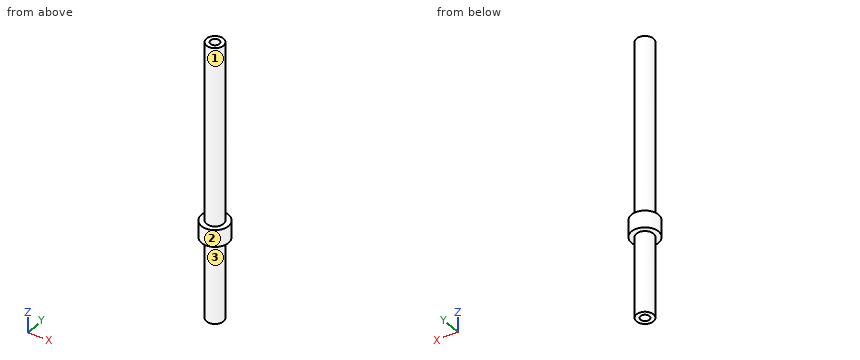
from build123d import *

# Parameters (mm, degrees)
SKETCH1_R                 = 2.5
BOSS_EXTRUDE1_DEPTH       = 24
SKETCH2_R                 = 4
BOSS_EXTRUDE2_DEPTH       = 5
SKETCH3_R                 = 2.5
BOSS_EXTRUDE3_DEPTH       = 53
M3X0_5_TAPPED_HOLE1_D     = 2.6
M3X0_5_TAPPED_HOLE1_DEPTH = 8
M3X0_5_TAPPED_HOLE1_TIP   = 0.781118805
M3X0_5_TAPPED_HOLE2_D     = 2.6
M3X0_5_TAPPED_HOLE2_DEPTH = 8
M3X0_5_TAPPED_HOLE2_TIP   = 0.781118805


with BuildPart() as part:
    # Sketch1 → Boss-Extrude1 (new body)
    with BuildSketch(Plane.XY):
        Circle(SKETCH1_R)
    extrude(amount=BOSS_EXTRUDE1_DEPTH)

    # Sketch2 → Boss-Extrude2 (add)
    with BuildSketch(Plane.XY.offset(24)):
        Circle(SKETCH2_R)
    extrude(amount=BOSS_EXTRUDE2_DEPTH)

    # Sketch3 → Boss-Extrude3 (add)
    with BuildSketch(Plane.XY.offset(29)):
        Circle(SKETCH3_R)
    extrude(amount=BOSS_EXTRUDE3_DEPTH)

    # M3x0.5 Tapped Hole1
    with Locations(Plane.XY.offset(82)):
        with Locations((0, 0)):
            Hole(M3X0_5_TAPPED_HOLE1_D / 2, depth=M3X0_5_TAPPED_HOLE1_DEPTH)
            with Locations((0, 0, -(M3X0_5_TAPPED_HOLE1_DEPTH + M3X0_5_TAPPED_HOLE1_TIP / 2))):  # 118° drill point
                Cone(0, M3X0_5_TAPPED_HOLE1_D / 2, M3X0_5_TAPPED_HOLE1_TIP, mode=Mode.SUBTRACT)

    # M3x0.5 Tapped Hole2
    with Locations(Plane(origin=(0, 0, 0), x_dir=(-1, 0, 0), z_dir=(0, 0, -1))):
        with Locations((0, 0)):
            Hole(M3X0_5_TAPPED_HOLE2_D / 2, depth=M3X0_5_TAPPED_HOLE2_DEPTH)
            with Locations((0, 0, -(M3X0_5_TAPPED_HOLE2_DEPTH + M3X0_5_TAPPED_HOLE2_TIP / 2))):  # 118° drill point
                Cone(0, M3X0_5_TAPPED_HOLE2_D / 2, M3X0_5_TAPPED_HOLE2_TIP, mode=Mode.SUBTRACT)


solid = part.part
CAD build for the part. Positions are in the model's coordinates, mm. Face numbers are marked on the shaded views. A direction names the side the tool comes from. Round coordinates to 2 decimals unless told otherwise and drop trailing zeros. Loops run counter-clockwise (first coordinate to the right, second up) from the corner with the lowest first, then second, coordinate; pieces in that order, holes last.
(1) Cut at A-A (z = 30). Give the cut face in (x, y).
(2) Which spindle directions (+Z, -Z, +X, -X, +Y, -Y) get a long thin tool onto all of the face, cutting with end or side? Do the marked faces 1, 2 and 3. Say none if no direction does.
(3) Drop flat-ended pins along their axis: pin 1 (1 mm diameter, centred on y = 1.5, z = 70.5, fed in from +X); pin 2 (2 mm diameter, centred on x = 0, y = 0, fed in from -Z); pin 3 (1.5 mm diameter, centred on x = 0, z = 68, fed in from -Y). Give the stop position or say it passes through.
(4) Cut at B-B (y = 3.25). Give the cut face in (x, z).
(5) Wall check: line 1 along Y through (x, z) = (0, 4.5); line 2 along X through (y, z) = (-0.25, 52); line 3 along Z through (x, y) = (-3.25, -1.5). Give the ranges that are in metal, low to high.
Findings below:
1. outline: circle Ø5 at (0, 0)
2. face 1: +Z
2. face 2: +Z, -Z
2. face 3: -Z
3. pin 1: stops at x = 2.29
3. pin 2: stops at z = 8.18
3. pin 3: stops at y = -2.5
4. outline: (-2.33, 24) - (2.33, 24) - (2.33, 29) - (-2.33, 29) - close
5. line 1: y = -2.5 to -1.3, 1.3 to 2.5
5. line 2: x = -2.49 to 2.49
5. line 3: z = 24 to 29
